Autodesk Inventor part; units mm, degrees
ref_plane "YZ Plane" through (0, 0, 0) normal (1, 0, 0) x (0, 1, 0)
ref_plane "XZ Plane" through (0, 0, 0) normal (0, 1, 0) x (-1, 0, 0)
ref_plane "XY Plane" through (0, 0, 0) normal (0, 0, 1) x (1, 0, 0)
sketch "Sketch1" plane through (0, 0, 0) normal (0, 1, 0) x (-1, 0, 0)
  line L0 (65.2374, 90.5054) -> (-34.7626, 90.5054)
  line L1 (-34.7626, 90.5054) -> (-34.7626, -109.4946)
  line L2 (-34.7626, -109.4946) -> (65.2374, -109.4946)
  line L3 (65.2374, -109.4946) -> (65.2374, 90.5054)
  point P0 (0, 0)
  dimension "d0" = 200
  dimension "d1" = 100
extrude "Extrusion1" add sketch "Sketch1" along normal blind 100
sketch "Sketch2" plane through (0, 0, 0) normal (0, -1, 0) x (1, 0, 0)
  line L0 (17.7626, 73.5054) -> (-48.2374, 73.5054)
  line L1 (-48.2374, 73.5054) -> (-48.2374, -92.4946)
  line L2 (-48.2374, -92.4946) -> (17.7626, -92.4946)
  line L3 (17.7626, -92.4946) -> (17.7626, 73.5054)
  line L4 (34.7626, 90.5054) -> (34.7626, -109.4946)
  line L5 (-65.2374, 90.5054) -> (34.7626, 90.5054)
  line L6 (34.7626, -109.4946) -> (-65.2374, -109.4946)
  line L7 (-65.2374, -109.4946) -> (-65.2374, 90.5054)
  point P0 (0, 0)
  dimension "d4" = 17
  dimension "d5" = 17
  dimension "d6" = 17
  dimension "d7" = 17
extrude "Extrusion2" cut sketch "Sketch2" against normal blind 38 contours L3 L2 L1 L0
fillet "Fillet1" radius 6.35 8 edges at (-15.2374, 100, 90.5054) (34.7626, 100, -9.4946) (34.7626, 50, 90.5054) (-65.2374, 50, 90.5054) (-65.2374, 100, -9.4946) (-15.2374, 100, -109.4946) (34.7626, 50, -109.4946) (-65.2374, 50, -109.4946)
sketch "Sketch3" plane through (0, 100, 0) normal (0, 1, 0) x (1, 0, 0)
  line L0 (-42.3145, -85.4273) -> (-42.3145, -16.4468) construction
  line L1 (-42.3145, -16.4468) -> (96.9241, -16.4468) construction
  line L2 (96.9241, -16.4468) -> (96.9241, -85.4273) construction
  line L3 (96.9241, -85.4273) -> (-42.3145, -85.4273) construction
  line L4 (-41.4344, -82.2493) -> (-41.4344, -41.0812)
  line L5 (-41.4344, -41.0812) -> (-31.9002, -41.0812)
  spline S0 degree 2 poles (-31.9002, -41.0812) (-27.0598, -46.4595) (-21.3882, -50.0287) knots 0 0 0 1 1 1
  spline S1 degree 2 poles (-21.3882, -50.0287) (-14.5432, -54.3802) (-6.1335, -56.9226) knots 0 0 0 1 1 1
  spline S2 degree 2 poles (-6.1335, -56.9226) (0.4181, -58.9272) (9.3656, -59.6117) knots 0 0 0 1 1 1
  line L6 (9.3656, -59.6117) -> (9.3656, -73.693)
  spline S3 degree 2 poles (9.3656, -73.693) (-3.0533, -72.0306) (-19.9214, -64.8922) (-29.5045, -57.1671) knots 0 0 0 1 2 2 2
  line L7 (-29.5045, -57.1671) -> (-29.5045, -82.2493)
  line L8 (-29.5045, -82.2493) -> (-41.4344, -82.2493)
  line L9 (-41.4344, -34.8718) -> (-41.4344, 6.2962)
  line L10 (-41.4344, 6.2962) -> (-31.9002, 6.2962)
  spline S4 degree 2 poles (-31.9002, 6.2962) (-27.0598, 0.918) (-21.3882, -2.6512) knots 0 0 0 1 1 1
  spline S5 degree 2 poles (-21.3882, -2.6512) (-14.5432, -7.0027) (-6.1335, -9.5451) knots 0 0 0 1 1 1
  spline S6 degree 2 poles (-6.1335, -9.5451) (0.4181, -11.5498) (9.3656, -12.2343) knots 0 0 0 1 1 1
  line L11 (9.3656, -12.2343) -> (9.3656, -26.3155)
  spline S7 degree 2 poles (9.3656, -26.3155) (-3.0533, -24.6531) (-19.9214, -17.5147) (-29.5045, -9.7896) knots 0 0 0 1 2 2 2
  line L12 (-29.5045, -9.7896) -> (-29.5045, -34.8718)
  line L13 (-29.5045, -34.8718) -> (-41.4344, -34.8718)
  line L14 (-41.4344, 17.9817) -> (-41.4344, 51.4246)
  line L15 (-41.4344, 51.4246) -> (-30.189, 51.4246)
  line L16 (-30.189, 51.4246) -> (-30.189, 28.7871)
  line L17 (-30.189, 28.7871) -> (-22.5616, 27.6137)
  spline S8 degree 2 poles (-22.5616, 27.6137) (-23.6373, 29.9605) (-24.7618, 34.5565) (-24.7618, 36.8056) knots 0 0 0 1 2 2 2
  spline S9 degree 2 poles (-24.7618, 36.8056) (-24.7618, 44.384) (-15.521, 53.8693) (-8.5293, 53.8693) knots 0 0 0 1 2 2 2
  spline S10 degree 2 poles (-8.5293, 53.8693) (-3.64, 53.8693) (5.4541, 48.98) (10.2457, 40.0325) (10.2457, 33.0408) knots 0 0 0 1 2 3 3 3
  spline S11 degree 2 poles (10.2457, 33.0408) (10.2457, 28.0048) (8.3388, 20.8664) (4.5741, 15.8304) (-0.2175, 12.7012) (-3.7867, 11.6745) knots 0 0 0 1 2 3 4 4 4
  line L18 (-3.7867, 11.6745) -> (-5.3512, 25.9513)
  spline S12 degree 2 poles (-5.3512, 25.9513) (-1.9287, 26.4891) (1.6405, 30.2539) (1.6405, 32.8941) knots 0 0 0 1 2 2 2
  spline S13 degree 2 poles (1.6405, 32.8941) (1.6405, 35.8277) (-2.8088, 39.6414) (-7.2581, 39.6414) knots 0 0 0 1 2 2 2
  spline S14 degree 2 poles (-7.2581, 39.6414) (-11.8051, 39.6414) (-16.01, 35.7788) (-16.01, 32.6008) knots 0 0 0 1 2 2 2
  spline S15 degree 2 poles (-16.01, 32.6008) (-16.01, 30.5473) (-14.9832, 28.6404) knots 0 0 0 1 1 1
  spline S16 degree 2 poles (-14.9832, 28.6404) (-14.2987, 27.2714) (-12.3919, 25.5601) knots 0 0 0 1 1 1
  line L19 (-12.3919, 25.5601) -> (-14.1031, 13.5324)
  line L20 (-14.1031, 13.5324) -> (-41.4344, 17.9817)
  line L21 (-2.0265, 60.2254) -> (-3.7867, 74.2577)
  spline S17 degree 2 poles (-3.7867, 74.2577) (-0.8531, 74.7956) (1.5916, 77.4358) (1.5916, 79.3426) knots 0 0 0 1 2 2 2
  spline S18 degree 2 poles (1.5916, 79.3426) (1.5916, 82.7652) (-1.8309, 84.672) knots 0 0 0 1 1 1
  spline S19 degree 2 poles (-1.8309, 84.672) (-4.3734, 86.041) (-12.5874, 86.7255) knots 0 0 0 1 1 1
  spline S20 degree 2 poles (-12.5874, 86.7255) (-9.9961, 84.1831) (-7.5514, 78.8537) (-7.5514, 75.3823) knots 0 0 0 1 2 2 2
  spline S21 degree 2 poles (-7.5514, 75.3823) (-7.5514, 68.5372) (-17.2323, 59.1498) (-24.664, 59.1498) knots 0 0 0 1 2 2 2
  spline S22 degree 2 poles (-24.664, 59.1498) (-29.7489, 59.1498) (-38.0608, 63.9413) (-42.3145, 72.302) (-42.3145, 78.6581) knots 0 0 0 1 2 3 3 3
  spline S23 degree 2 poles (-42.3145, 78.6581) (-42.3145, 86.2855) (-37.0829, 95.4774) (-25.6908, 101.0023) (-16.3033, 101.0023) knots 0 0 0 1 2 3 3 3
  spline S24 degree 2 poles (-16.3033, 101.0023) (-2.5643, 101.0023) (10.2457, 89.4146) (10.2457, 79.196) knots 0 0 0 1 2 2 2
  spline S25 degree 2 poles (10.2457, 79.196) (10.2457, 73.1332) (7.4588, 66.0926) (2.0316, 61.4966) (-2.0265, 60.2254) knots 0 0 0 1 2 3 3 3
  spline S26 degree 2 poles (-24.7129, 86.1877) (-28.82, 86.1877) (-33.5137, 82.0318) (-33.5137, 79.0493) knots 0 0 0 1 2 2 2
  spline S27 degree 2 poles (-33.5137, 79.0493) (-33.5137, 76.2624) (-29.3089, 72.5465) (-25.0552, 72.5465) knots 0 0 0 1 2 2 2
  spline S28 degree 2 poles (-25.0552, 72.5465) (-20.8015, 72.5465) (-16.3033, 76.409) (-16.3033, 79.2937) knots 0 0 0 1 2 2 2
  spline S29 degree 2 poles (-16.3033, 79.2937) (-16.3033, 82.2762) (-20.6548, 86.1877) (-24.7129, 86.1877) knots 0 0 0 1 2 2 2
  point P0 (0, 0)
extrude "Extrusion3" cut sketch "Sketch3" against normal blind 12.8
properties part number "7759Block"
CAD build for the part. Positions are in the model's coordinates, mm. A direction names the side the tool comes from. Give positions to 0.01 mm unless a question says otherwise; leave off trailing zeros. Order: outer loops, then holes, each group sorted by start corner. A loop starts at its lowest first (then second) coordinate and runs counter-clockwise, first axis right, second up. Notation, with made-up numbers: (-9.5, 43.25) -> (31.5, 43.25) arc R21 cw to (31.5, 67.25) -> close; hole circle Ø7 at (75.25, -4). An arc over 180 degrees is marked (long way). Return JSON: item names as keys, results as strings.
Q1. Which spindle directions (+Z, -Z, +X, -X, +Y, -Y) get a long thin tool onto all of the face, cutting with end or side? Do faces 1 (the face through (-36, 94, -51.425)), 2 (the face through (-16, 46, 90.505)), 3 (the face through (17.763, 19, -11)). Say none if no direction does.
Working result:
{"face 1": "+Y", "face 2": "+Z, +X, -X, +Y, -Y", "face 3": "-Y"}
Q2. Drill centre lines: line 1 (X direction, y = 93, z = -62); line 2 (X direction, y = 25.5, z = -66); line 3 (Y direction, x = -5.5, z = -36.5). Where is each one in solid material? Low to high.
Working result:
{"line 1": "-65.24 to -34.65, -14.66 to -2.25, 2.15 to 34.76", "line 2": "-65.24 to -48.24, 17.76 to 34.76", "line 3": "38 to 100"}
Q3. Saw through at A-A (y = 20). Write the cut outline in (x, z), then the cut area to 3 significant figures.
Working result:
{"outline": "(-65.24, -103.14) arc R6.35 ccw to (-58.89, -109.49) -> (28.41, -109.49) arc R6.35 ccw to (34.76, -103.14) -> (34.76, 84.16) arc R6.35 ccw to (28.41, 90.51) -> (-58.89, 90.51) arc R6.35 ccw to (-65.24, 84.16) -> close; hole (-48.24, -92.49) -> (17.76, -92.49) -> (17.76, 73.51) -> (-48.24, 73.51) -> close", "area": "9,010 mm²"}
Q4. Saw through at C-C (z = 31.5). Write the cut outline in (x, y).
Working result:
{"outline": "(-65.24, 0) -> (-48.24, 0) -> (-48.24, 38) -> (17.76, 38) -> (17.76, 0) -> (34.76, 0) -> (34.76, 93.65) arc R6.35 ccw to (28.41, 100) -> (-29.5, 100) -> (-29.5, 87.2) -> (-41.43, 87.2) -> (-41.43, 100) -> (-58.89, 100) arc R6.35 ccw to (-65.24, 93.65) -> close"}
Q5. Saw through at B-B (x = 15). Write the cut outline in (y, z).
Working result:
{"outline": "(0, -109.49) -> (93.65, -109.49) arc R6.35 ccw to (100, -103.14) -> (100, 84.16) arc R6.35 ccw to (93.65, 90.51) -> (0, 90.51) -> (0, 73.51) -> (38, 73.51) -> (38, -92.49) -> (0, -92.49) -> close"}
Q6. Flat gauge pins, fed straight in: pin 1 (20.5 mm diameter, centred on x = -23, z = 12.5, fed in from +Y); pin 2 (6 mm diameter, centred on x = 8, z = -10, fed in from -Y). Where does each tip first touch, or does it go through?
Working result:
{"pin 1": "y = 100", "pin 2": "y = 38"}
Q7. Mould opens along X. For faces 4 (the face through (-16, 38, -8)), 5 (the face through (32.952, 47.481, -107.585)), 6 (the face through (19, 0, -8)) say: pulls with the +X half, pulls with the -X half, needs draft (parallel to the pull), parting line crosses it, or undercut.
Working result:
{"face 4": "undercut", "face 5": "pulls with the +X half", "face 6": "needs draft"}
